Read the model definition and answer for the solid it produces. Units are mm, in the model's axes. A direction names the side the tool comes from. Coordinates: 2 decimals unless noted, no trailing zeros. Loops run counter-clockwise (first coordinate to the right, second up) from the corner with the lowest first, then second, coordinate; pieces in that order, holes last.
from build123d import *

# Parameters (mm, degrees)
SKETCH1_R             = 3
MOTORANDGEARBOX_DEPTH = 26.9
ENCODER_START         = 4.2
SKETCH2_R             = 3
ENCODER_DEPTH         = 4.2
SKETCH3_R             = 2
BOSS_EXTRUDE3_DEPTH   = 0.5
SKETCH4_R             = 1
BOSS_EXTRUDE4_DEPTH   = 0.8
SKETCH5_R             = 0.75
BOSS_EXTRUDE5_DEPTH   = 4.1
SKETCH6_OUTSIDE_W     = 15.494
SKETCH6_OUTSIDE_H     = 15.494
CUT_EXTRUDE1_DEPTH    = 3


with BuildPart() as part:
    # Sketch1 → motorAndGearbox (new body)
    with BuildSketch(Plane(origin=(0, 0, 0), x_dir=(1, 0, 0), z_dir=(0, 1, 0))):
        with Locations(Location((0, 0, 0), (0, 0, 90))):
            Circle(SKETCH1_R)
    extrude(amount=MOTORANDGEARBOX_DEPTH)

    # Sketch2 → encoder (add)
    with BuildSketch(Plane.XZ.offset(ENCODER_START)):
        with Locations(Location((0, 0, 0), (0, 0, 270))):
            Circle(SKETCH2_R)
    extrude(amount=-ENCODER_DEPTH)

    # Sketch3 → Boss-Extrude3 (add)
    with BuildSketch(Plane(origin=(0, 26.9, 0), x_dir=(1, 0, 0), z_dir=(0, 1, 0))):
        with Locations(Location((0, 0, 0), (0, 0, 270))):
            Circle(SKETCH3_R)
    extrude(amount=BOSS_EXTRUDE3_DEPTH)

    # Sketch4 → Boss-Extrude4 (add)
    with BuildSketch(Plane(origin=(0, 27.4, 0), x_dir=(1, 0, 0), z_dir=(0, 1, 0))):
        with Locations(Location((0, 0, 0), (0, 0, 270))):
            Circle(SKETCH4_R)
    extrude(amount=BOSS_EXTRUDE4_DEPTH)

    # Sketch5 → Boss-Extrude5 (add)
    with BuildSketch(Plane(origin=(0, 28.2, 0), x_dir=(1, 0, 0), z_dir=(0, 1, 0))):
        with Locations(Location((0, 0, 0), (0, 0, 270))):
            Circle(SKETCH5_R)
    extrude(amount=BOSS_EXTRUDE5_DEPTH)

    # Sketch6 outside → Cut-Extrude1 (cut)
    with BuildSketch(Plane(origin=(0, 32.3, 0), x_dir=(1, 0, 0), z_dir=(0, 1, 0))):
        Rectangle(SKETCH6_OUTSIDE_W, SKETCH6_OUTSIDE_H)
        with BuildLine():
            Line((-0.509901951, -0.55), (0.509901951, -0.55))
            ThreePointArc((0.509901951, -0.55), (0, 0.75), (-0.509901951, -0.55))
        make_face(mode=Mode.SUBTRACT)
    extrude(amount=-CUT_EXTRUDE1_DEPTH, mode=Mode.SUBTRACT)


solid = part.part
Item 1: A cutting plane is placed at A-A on z = 0. Determine the outline of the cut face in (x, y), then the cut area to 3 significant figures.
Numbers:
outline: (-3, -4.2) - (3, -4.2) - (3, 26.9) - (2, 26.9) - (2, 27.4) - (1, 27.4) - (1, 28.2) - (0.75, 28.2) - (0.75, 32.3) - (-0.75, 32.3) - (-0.75, 28.2) - (-1, 28.2) - (-1, 27.4) - (-2, 27.4) - (-2, 26.9) - (-3, 26.9) - close
area: 196 mm2
Item 2: A cutting plane is placed at C-C on y = 29. Determine the outline of the cut face in (x, z), then the cut area to 3 significant figures.
Numbers:
outline: circle Ø1.5 at (0, 0)
area: 1.77 mm2
Item 3: A cutting plane is placed at B-B on x = 0. Determine the outline of the cut face in (y, z).
Numbers:
outline: (-4.2, -3) - (26.9, -3) - (26.9, -2) - (27.4, -2) - (27.4, -1) - (28.2, -1) - (28.2, -0.75) - (32.3, -0.75) - (32.3, 0.55) - (29.3, 0.55) - (29.3, 0.75) - (28.2, 0.75) - (28.2, 1) - (27.4, 1) - (27.4, 2) - (26.9, 2) - (26.9, 3) - (-4.2, 3) - close
Item 4: Which of the six approach directions +Z, -Z, +X, -X, +Y, -Y give full straight-line access (tool end or side, diameter ignored) to faces 1 (the face through (0, -4.2, 0)), 2 (the face through (-1.952, 27.146, -0.434)), 3 (the face through (0, 31, 0.55))?
Numbers:
face 1: +Z, -Z, +X, -X, -Y
face 2: +Y
face 3: +Z, +X, -X, +Y
Item 5: A cutting plane is placed at D-D on z = 1.6. Determine the outline of the cut face in (x, y).
Numbers:
outline: (-2.54, -4.2) - (2.54, -4.2) - (2.54, 26.9) - (1.2, 26.9) - (1.2, 27.4) - (-1.2, 27.4) - (-1.2, 26.9) - (-2.54, 26.9) - close
Item 6: Given pin 1 (3 mm diameter, centred on x = 1, y = 3, fed in from +Z); pin 2 (1.5 mm diameter, centred on y = 13, z = 2, fed in from -X); pin 3 (1.1 mm diameter, centred on x = 0, y = 31.5, fed in from +Z), each flat-ended and moving along its own axis, determine where each tip first touches the part or whether it passes through.
Numbers:
pin 1: stops at z = 3
pin 2: stops at x = -2.73
pin 3: stops at z = 0.55
Item 7: Find the intervals of material crossed by line 1 along Y through (x, z) = (1.05, -2.65); line 2 along Z through (x, y) = (0.1, 26); line 3 along Y through (x, z) = (0.85, 1), in increasing order.
Numbers:
line 1: y = -4.2 to 26.9
line 2: z = -3 to 3
line 3: y = -4.2 to 27.4
